Verification items for the finished model (mm, model axes). Coordinates: 2 decimals unless noted, no trailing zeros. Loops run counter-clockwise (first coordinate to the right, second up) from the corner with the lowest first, then second, coordinate; pieces in that order, holes last. Notation, with made-up numbers: (71, 35.25) - (90, 35.25) arc R29 ccw to (90, 63.25) - close; hole circle Ø7 at (89.25, -18). An arc over 180 degrees is marked (long way). Answer as CSV lines item,"result". Start each with the question number.
1. Cross-section at A-A (y = -146.5). Enter the section's corners in (x, z), plus the area to 3 significant figures.
2. Gauge pin test, flat end, axial feed: P1, Ø1, axis at x = -142, z = 15.5, coming from the +Y side. Record the tip position at first contact, or that the pin passes through.
3. Material ranges on line 1 (Y direction, x = 155, z = 6.75); line 2 (X direction, y = -116.5, z = 12.75); line 3 (Y direction, x = 171.5, z = 1), recorded low to high. Write a range as [from, to].
4. Release check for a two-part mould opening along Y. For faces 1 (the flat face through (-3, 2, 19)), 2 (the flat face through (28, 175, 9)), 3 (the cylindrical face through (127.99, -127.09, 9.63)) record: pulls with the +Y half, pulls with the -Y half, needs draft (parallel to the pull), parting line crosses it, or undercut.
```python
from build123d import *

# Parameters (mm, degrees)
F0_W     = 400
F0_H     = 350
F1_DEPTH = 19
F3_DEPTH = 19.001
F4_R     = 28.6407244268
F5_DEPTH = 19.0010001


with BuildPart() as f1:
    # F0 (on Top) → F1 (new body)
    with BuildSketch(Plane.XY):
        Rectangle(F0_W, F0_H)
    extrude(amount=F1_DEPTH)

    # F2 (on face) → F3 (cut, through all)
    with BuildSketch(Plane.XY.offset(19)):
        with BuildLine():
            add(Edge.make_bspline(
                [(-140, 175), (-157.942733111, 173.3225620191), (-189.2184929725, 165.8035915867), (-198.0018895699, 132.3529522536), (-200, 115)],
                knots=[0, 0, 0, 0, 0.4965617875, 1, 1, 1, 1], degree=3))
            Line((-140, 175), (-200, 175))
            Line((-200, 175), (-200, 115))
        make_face()
    extrude(amount=-F3_DEPTH, mode=Mode.SUBTRACT)

    # F4 (on face) → F5 (cut, through all)
    with BuildSketch(Plane.XY.offset(19)):
        with Locations((156.6020158332, -128.344308295)):
            Circle(F4_R)
    extrude(amount=-F5_DEPTH, mode=Mode.SUBTRACT)


solid = f1.part
```
Values follow:
1,outline,"(-200, 0) - (134.45, 0) - (134.45, 19) - (-200, 19) - close; (178.75, 0) - (200, 0) - (200, 19) - (178.75, 19) - close"
1,area,"6,760 mm²"
2,P1,"stops at y = 174.85"
3,line 1,"y = [-175, -156.94], [-99.75, 175]"
3,line 2,"x = [-200, 130.53], [182.68, 200]"
3,line 3,"y = [-175, -152.81], [-103.88, 175]"
4,face 1,"needs draft"
4,face 2,"pulls with the +Y half"
4,face 3,"undercut"
